For this review, take the finished solid that the model builds, in its own axes (mm). Face numbers are marked on the shaded views. A direction names the side the tool comes from. Coordinates: 2 decimals unless noted, no trailing zeros. Order: outer loops, then holes, each group sorted by start corner. A loop starts at its lowest first (then second) coordinate and runs counter-clockwise, first axis right, second up. Notation, with made-up numbers: M 39.25,22.5 L 48.25,22.5 A37 cw 48.25,58.5 Z; hole C -18,30.5 d8. An arc over 180 degrees is marked long. Use CSV: the item, a comma, the result in double quotes.
```python
from build123d import *

# Parameters (mm, degrees)
BOSS_EXTRUDE1_DEPTH = 10
FILLET1_R           = 2


with BuildPart() as part:
    # Sketch1 → Boss-Extrude1 (new, symmetric)
    with BuildSketch(Plane(origin=(0, 0, 0), x_dir=(1, 0, 0), z_dir=(0, 1, 0))):
        with BuildLine():
            Line((4, -79.806298407), (4, -100))
            Line((4, -100), (0, -100))
            Line((0, -100), (0, -79.806298407))
            ThreePointArc((0, -79.806298407), (4.930609057, -58.155663313), (18.75, -40.775060917))
            ThreePointArc((18.75, -40.775060917), (24.661331748, -0.273616166), (-15.333333333, 8.429121051))
            ThreePointArc((-15.333333333, 8.429121051), (-30.097999134, 2.145645207), (-46, 0))
            Line((-46, 0), (-46, 4))
            ThreePointArc((-46, 4), (-31.158132525, 6.002602194), (-17.377777778, 11.867179648))
            ThreePointArc((-17.377777778, 11.867179648), (27.949509314, 2.004077469), (21.25, -43.897559916))
            ThreePointArc((21.25, -43.897559916), (8.536160332, -59.88771412), (4, -79.806298407))
        make_face()
    extrude(amount=BOSS_EXTRUDE1_DEPTH, both=True)

    # Fillet1
    fillet1_edges = [part.edges().sort_by_distance(p)[0] for p in [
        (0, -10, 89.903149204),
        (4.930609057, -10, 58.155663313),
        (24.661331748, -10, 0.273616166),
        (4, -10, 89.903149204),
        (8.536160332, -10, 59.88771412),
        (27.949509314, -10, -2.004077469),
        (0, 10, 89.903149204),
        (4.930609057, 10, 58.155663313),
        (24.661331748, 10, 0.273616166),
        (4, 10, 89.903149204),
        (8.536160332, 10, 59.88771412),
        (27.949509314, 10, -2.004077469),
        (-30.097999134, -10, -2.145645207),
        (-31.158132525, -10, -6.002602194),
        (-30.097999134, 10, -2.145645207),
        (-31.158132525, 10, -6.002602194),
    ]]
    fillet(fillet1_edges, radius=FILLET1_R - 0.0001)  # a hair under: the kernel refuses the full size


solid = part.part
```
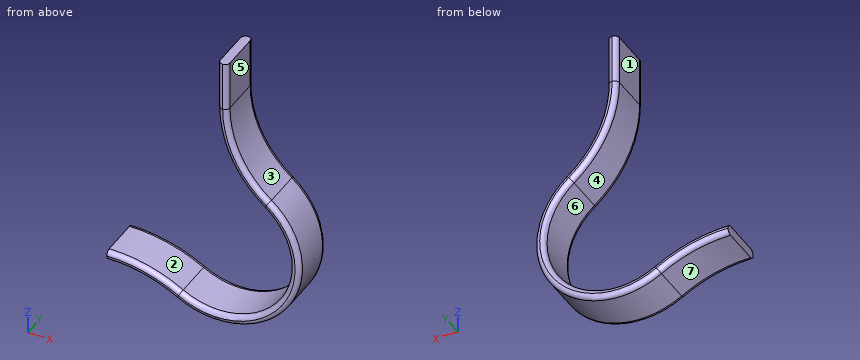
Item 1: Add section A-A on y = 0.75. State the section outline as (x, z) points, and give its area (3 significant figures).
Solutions:
outline,"M -46,-4 A56 cw -17.38,-11.87 A34 ccw 21.25,43.9 A46 cw 4,79.81 L 4,100 L 0,100 L 0,79.81 A50 ccw 18.75,40.78 A30 cw -15.33,-8.43 A60 ccw -46,0 Z"
area,"762 mm^2"
Item 2: For the marked faces 1, 2, 3 and 4, list the 3-axis set-ups (+Z, -Z, +X, -X, +Y, -Y) from which the entire face can be reached by the end or side of a thin tool; tool diameter is ignored.
Solutions:
face 1,"+Z, -X, +Y, -Y"
face 2,"+Z, +Y, -Y"
face 3,"+Z, +X, +Y, -Y"
face 4,"-X, +Y, -Y"
Item 3: To check wall thickness, follow line 1 along X through (y, z) = (0.25, 82); line 2 along Y through (x, z) = (4.5, 65); line 3 along Z through (x, y) = (14, 1.5). State the ranges of each line that lie inside material, in increasing order. Write a range as [from, to].
Solutions:
line 1,"[0, 4]"
line 2,"[-9.99, 9.99]"
line 3,"[-13.63, -9.18], [45.11, 51.17]"
Item 4: Clearance check with flat-ended pins moving along their axes: pin 1 Ø2 at (x, y) = (20.5, -6) entering from +Z; pin 2 Ø5 at (y, z) = (-8, 49.5) entering from -X; pin 3 Ø5 at (y, z) = (-2, 86) entering from +X. State where each tip first meets the part, or that it passes through.
Solutions:
pin 1,"z = 45.37"
pin 2,"x = 8.45"
pin 3,"x = 4"
Item 5: Draft analysis for pull direction X (two halves, no side actions). For the marked faces 5, 6 and 7, state which applies: released by +X, released by -X, zero draft, split by the parting line, or undercut.
Solutions:
face 5,"released by +X"
face 6,"undercut"
face 7,"released by -X"
